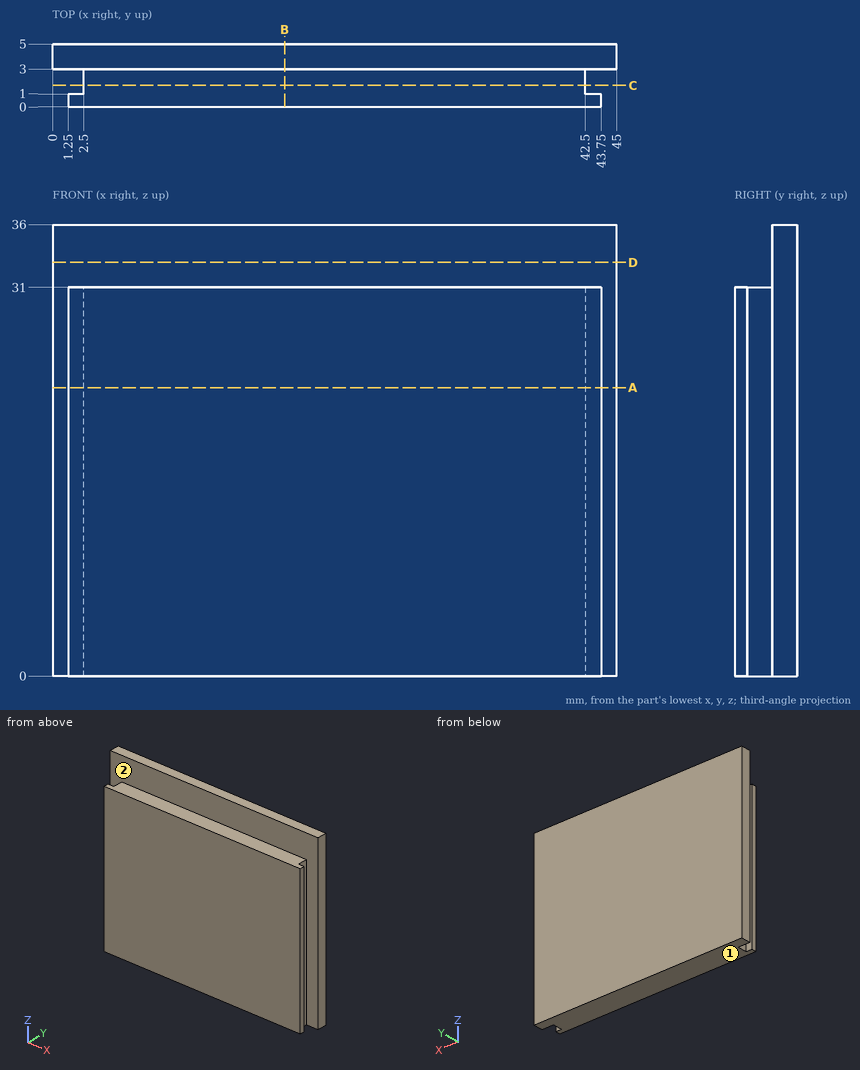
Here's the drawing with two shaded views (mm, measured from the low corner). I have some questions. A direction names the side the tool comes from. Coordinates: 2 decimals unless noted, no trailing zeros. Order: outer loops, then holes, each group sorted by start corner. A loop starts at its lowest first (then second) coordinate and runs counter-clockwise, first axis right, second up. Notation, with made-up numbers: (-19.75, 46) - (7.25, 46) arc R13 cw to (7.25, 53) - close; hole circle Ø7 at (-12, 55.5). An arc over 180 degrees is marked (long way). Use CSV: the item, a comma, the result in double quotes. Start each with the question number.
1. Suppose I cut it at B-B on x = 18.5. List the corners of the cut face in (y, z) for me, then the cut area to 3 significant figures.
2. I'm going to push flat-ended pins straight in: pin 1 (0.8 mm diameter, centred on y = 0.5, z = 21, fed in from +X); pin 2 (1 mm diameter, centred on y = 2, z = 22.5, fed in from +X); pin 3 (1.1 mm diameter, centred on y = 0.5, z = 10.5, fed in from -X). Where does each tip first touch, or does it pass through?
3. Please list where these lines run through material, in increasing order: line 1 (X direction, y = 1.55, z = 20); line 2 (Z direction, x = 34.5, y = 2.3); line 3 (Y direction, x = 21, z = 32.5). Write a range as from..to.
4. Suppose I cut it at D-D on z = 33. List the corners of the cut face in (x, y) for me, then the cut area to 3 significant figures.
5. Suppose I cut it at A-A on z = 23. List the corners of the cut face in (x, y) for me, then the cut area to 4 significant figures.
6. Suppose I cut it at C-C on y = 1.7. List the corners of the cut face in (x, z) for me, then the cut area to 3 significant figures.
7. For the marked faces 1 and 2, which set-ups out of +Z, -Z, +X, -X, +Y, -Y let a thin tool reach every point of the face, with its end or its side?
Output:
1,outline,"(0, 0) - (5, 0) - (5, 36) - (3, 36) - (3, 31) - (0, 31) - close"
1,area,"165 mm2"
2,pin 1,"stops at x = 43.75"
2,pin 2,"stops at x = 42.5"
2,pin 3,"stops at x = 1.25"
3,line 1,"x = 2.5..42.5"
3,line 2,"z = 0..31"
3,line 3,"y = 3..5"
4,outline,"(0, 3) - (45, 3) - (45, 5) - (0, 5) - close"
4,area,"90.0 mm2"
5,outline,"(0, 3) - (2.5, 3) - (2.5, 1) - (1.25, 1) - (1.25, 0) - (43.75, 0) - (43.75, 1) - (42.5, 1) - (42.5, 3) - (45, 3) - (45, 5) - (0, 5) - close"
5,area,"212.5 mm2"
6,outline,"(2.5, 0) - (42.5, 0) - (42.5, 31) - (2.5, 31) - close"
6,area,"1,240 mm2"
7,face 1,"-Z, +X, -X, +Y, -Y"
7,face 2,"+Z"
